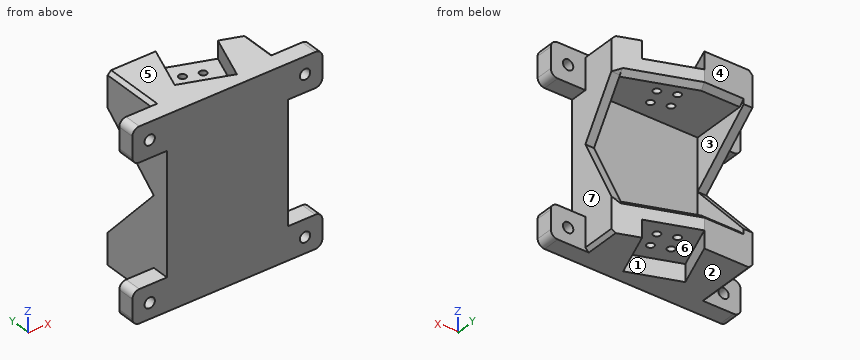
```python
from build123d import *

# Parameters (mm, degrees)
EXTRUDE_1_DEPTH          = 35
EXTRUDE_1_2_DEPTH        = 35
CUT_EXTRUDE_1_DEPTH      = 104.662915259
CUT_EXTRUDE_1_DEPTH_BACK = 104.662915259
SKETCH_2_R               = 2.1
SKETCH_3_W               = 70
SKETCH_3_H               = 10
EXTRUDE_2_DEPTH          = 89
EXTRUDE_3_DEPTH          = 10
EXTRUDE_4_DEPTH          = 10
SKETCH_8_W               = 20
SKETCH_8_H               = 19
SKETCH_8_R               = 3
SKETCH_8_H_2             = 20
EXTRUDE_9_DEPTH          = 10
EXTRUDE_10_DEPTH         = 5
CUT_EXTRUDE_2_DEPTH      = 130.251692445
CUT_EXTRUDE_2_DEPTH_BACK = 130.251692445
EXTRUDE_12_DEPTH         = 5
FILLET_1_R               = 4
FILLET_2_R               = 4
CHAMFER_3_SIZE           = 3
CHAMFER_4_SIZE           = 2


with BuildPart() as part:
    # Sketch 1 → Extrude 1 (new body)
    with BuildSketch(Plane(origin=(0, 0, 0), x_dir=(1, 0, 0), z_dir=(0, 1, 0))):
        Polygon((0, -40), (30, -40), (30, -30), (-40, -30), (-40, -40), align=None)
    extrude(amount=EXTRUDE_1_DEPTH)


with BuildPart() as body_2:
    # Sketch 1 → Extrude 1 2 (new body)
    with BuildSketch(Plane(origin=(0, 0, 0), x_dir=(1, 0, 0), z_dir=(0, 1, 0))):
        Polygon((0, 49), (30, 49), (30, 39), (-40, 39), (-40, 49), align=None)
    extrude(amount=EXTRUDE_1_2_DEPTH)


with BuildPart() as cut_extrude_1_tool:
    # Sketch 2 → Cut-Extrude 1 (new, two sides: drawn at the far end of the back side and taken through both)
    with BuildSketch(Plane.XY.offset(40).offset(-CUT_EXTRUDE_1_DEPTH_BACK)):
        with Locations((0, 10)):
            Circle(SKETCH_2_R)
        with Locations((-9.396926208, 13.420201433)):
            Circle(SKETCH_2_R)
        with Locations((3.420201433, 19.396926208)):
            Circle(SKETCH_2_R)
        with Locations((-5.976724775, 22.817127641)):
            Circle(SKETCH_2_R)
    extrude(amount=CUT_EXTRUDE_1_DEPTH + CUT_EXTRUDE_1_DEPTH_BACK)


with BuildPart() as part_1:
    add(part.part)

    # Cut-Extrude 1: cut by cut_extrude_1_tool
    add(cut_extrude_1_tool.part, mode=Mode.SUBTRACT)



with BuildPart() as body_2_1:
    add(body_2.part)

    # Cut-Extrude 1: cut by cut_extrude_1_tool
    add(cut_extrude_1_tool.part, mode=Mode.SUBTRACT)


with BuildPart() as part_2:
    add(part_1.part)

    add(body_2_1.part)  # Extrude 2 merges body 2
    # Sketch 3 → Extrude 2 (add)
    with BuildSketch(Plane.XY.offset(40)):
        with Locations((-5, -5)):
            Rectangle(SKETCH_3_W, SKETCH_3_H)
    extrude(amount=-EXTRUDE_2_DEPTH)

    # Sketch 4 → Extrude 3 (add)
    with BuildSketch(Plane.XY.offset(40)):
        Polygon((5.976724775, -2.817127641), (-22.214053849, 7.443476659), (-12.184299593, 35), (-40, 35), (-40, -10), (30, -10), (30, 35), (19.741033581, 35), align=None)
    extrude(amount=EXTRUDE_3_DEPTH)

    # Sketch 5 → Extrude 4 (add)
    with BuildSketch(Plane(origin=(0, 0, -49), x_dir=(-1, 0, 0), z_dir=(0, 0, -1))):
        Polygon((-30, 35), (-30, -10), (40, -10), (40, 35), (12.184299593, 35), (22.214053849, 7.443476659), (-5.976724775, -2.817127641), (-19.741033581, 35), align=None)
    extrude(amount=EXTRUDE_4_DEPTH)

    # Sketch 8 → Extrude 9 (add)
    # profile 1 of 4: a face of its own
    with BuildSketch(Plane(origin=(0, -10, 0), x_dir=(-1, 0, 0), z_dir=(0, -1, 0))):
        with Locations((-40, 49.5)):
            Rectangle(SKETCH_8_W, SKETCH_8_H)
        with Locations(Location((-40, 50, 0), (0, 0, 90))):
            Circle(SKETCH_8_R, mode=Mode.SUBTRACT)
    # profile 2 of 4: a face of its own
    with BuildSketch(Plane(origin=(0, -10, 0), x_dir=(-1, 0, 0), z_dir=(0, -1, 0))):
        with Locations((-40, -40)):
            Rectangle(SKETCH_8_W, SKETCH_8_H_2)
        with Locations(Location((-40, -40, 0), (0, 0, 90))):
            Circle(SKETCH_8_R, mode=Mode.SUBTRACT)
    # profile 3 of 4: a face of its own
    with BuildSketch(Plane(origin=(0, -10, 0), x_dir=(-1, 0, 0), z_dir=(0, -1, 0))):
        with Locations((50, 49.5)):
            Rectangle(SKETCH_8_W, SKETCH_8_H)
        with Locations(Location((50, 50, 0), (0, 0, 90))):
            Circle(SKETCH_8_R, mode=Mode.SUBTRACT)
    # profile 4 of 4: a face of its own
    with BuildSketch(Plane(origin=(0, -10, 0), x_dir=(-1, 0, 0), z_dir=(0, -1, 0))):
        with Locations((50, -40)):
            Rectangle(SKETCH_8_W, SKETCH_8_H_2)
        with Locations(Location((50, -40, 0), (0, 0, 90))):
            Circle(SKETCH_8_R, mode=Mode.SUBTRACT)
    extrude(amount=-EXTRUDE_9_DEPTH)

    # Sketch 6 → Extrude 10 (add)
    with BuildSketch(Plane.ZY.offset(40)):
        Polygon((-39, 0), (0, 0), (-39, 35), align=None)
        Polygon((30, 0), (30, 35), (0, 0), align=None)
    extrude(amount=-EXTRUDE_10_DEPTH)

    # Sketch 10 → Cut-Extrude 2 (cut, two sides: drawn at the far end of the back side and taken through both)
    with BuildSketch(Plane.XY.offset(50).offset(-CUT_EXTRUDE_2_DEPTH_BACK)):
        Polygon((30, 19.646170595), (-12.184299593, 35), (30, 35), align=None)
    extrude(amount=CUT_EXTRUDE_2_DEPTH + CUT_EXTRUDE_2_DEPTH_BACK, mode=Mode.SUBTRACT)

    # Sketch 9 → Extrude 12 (add)
    with BuildSketch(Plane(origin=(30, 0, 0), x_dir=(0, 0, -1), z_dir=(1, 0, 0))):
        Polygon((39, 19.646170595), (39, 0), (0, 0), align=None)
        Polygon((0, 0), (-30, 19.646170595), (-30, 0), align=None)
    extrude(amount=-EXTRUDE_12_DEPTH)

    # Fillet 1
    fillet_1_edges = [part_2.edges().sort_by_distance(p)[0] for p in [
        (50, -5, -59),
        (50, -5, 50),
        (-60, -5, -59),
        (-60, -5, 50),
    ]]
    fillet(fillet_1_edges, radius=FILLET_1_R)

    # Fillet 2
    fillet_2_edges = [part_2.edges().sort_by_distance(p)[0] for p in [
        (50, -5, -40),
        (50, -5, 30),
        (-60, -5, -40),
        (-60, -5, 30),
    ]]
    fillet(fillet_2_edges, radius=FILLET_2_R)

    # Chamfer 3
    # the kernel refuses this chamfer: 3 mm, written as the material it takes off along each edge
    with BuildSketch(Plane(origin=(-4.469250629, 35, -39), x_dir=(0, 0.027495876610586768, -0.9996219169112968), z_dir=(-1, 0, 0))) as chamfer_3_piece_1:
        Polygon((CHAMFER_3_SIZE * 0.999621916911, CHAMFER_3_SIZE * 0.0274958766106), (-CHAMFER_3_SIZE * 0.0274958766106, CHAMFER_3_SIZE * 0.999621916911), (0, 0), align=None)
    extrude(amount=30.530749371, mode=Mode.SUBTRACT)
    with BuildSketch(Plane(origin=(-19.434074173, 37.638702152, -39), x_dir=(0.009404143659217951, 0.02583767235300856, -0.9996219169112968), z_dir=(0.9396926207859079, -0.34202014332567027, 0))) as chamfer_3_piece_2_section:
        Polygon((CHAMFER_3_SIZE * 0.999621916911, -CHAMFER_3_SIZE * 0.0274958766106), (-CHAMFER_3_SIZE * 0.0274958766106, -CHAMFER_3_SIZE * 0.999621916911), (0, 0), align=None)
    chamfer_3_piece_2 = extrude(amount=60.321691902, mode=Mode.PRIVATE)
    chamfer_3_piece_2 = split(chamfer_3_piece_2, bisect_by=Plane(origin=(25, 27.771188546, -39.985901666), z_dir=(-1, 0, 0)), keep=Keep.TOP, mode=Mode.PRIVATE)
    add(chamfer_3_piece_2, mode=Mode.SUBTRACT)
    with BuildSketch(Plane(origin=(-19.434074173, 37.638702152, -39), x_dir=(0.009404143659217951, 0.02583767235300856, -0.9996219169112968), z_dir=(0.9396926207859079, -0.34202014332567027, 0))) as chamfer_3_piece_3_section:
        Polygon((CHAMFER_3_SIZE * 0.999621916911, -CHAMFER_3_SIZE * 0.0274958766106), (-CHAMFER_3_SIZE * 0.0274958766106, -CHAMFER_3_SIZE * 0.999621916911), (0, 0), align=None)
    chamfer_3_piece_3 = extrude(amount=60.321691902, mode=Mode.PRIVATE)
    chamfer_3_piece_3 = split(chamfer_3_piece_3, bisect_by=Plane(origin=(26.25970181, 20.183987428, -40.067630782), z_dir=(0, 0.8930842834154016, 0.4498893894241103)), keep=Keep.TOP, mode=Mode.PRIVATE)
    add(chamfer_3_piece_3, mode=Mode.SUBTRACT)
    with BuildSketch(Plane(origin=(-4.469250629, 35, 30), x_dir=(0, 0.027495876610586768, 0.9996219169112968), z_dir=(-1, 0, 0))) as chamfer_3_piece_4:
        Polygon((CHAMFER_3_SIZE * 0.999621916911, -CHAMFER_3_SIZE * 0.0274958766106), (-CHAMFER_3_SIZE * 0.0274958766106, -CHAMFER_3_SIZE * 0.999621916911), (0, 0), align=None)
    extrude(amount=30.530749371, mode=Mode.SUBTRACT)
    with BuildSketch(Plane(origin=(-19.434074173, 37.638702152, 30), x_dir=(0.009404143659217682, 0.025837672353007816, 0.9996219169112968), z_dir=(0.9396926207859079, -0.34202014332567027, 0))) as chamfer_3_piece_5_section:
        Polygon((CHAMFER_3_SIZE * 0.999621916911, CHAMFER_3_SIZE * 0.0274958766106), (-CHAMFER_3_SIZE * 0.0274958766106, CHAMFER_3_SIZE * 0.999621916911), (0, 0), align=None)
    chamfer_3_piece_5 = extrude(amount=60.321691902, mode=Mode.PRIVATE)
    chamfer_3_piece_5 = split(chamfer_3_piece_5, bisect_by=Plane(origin=(25, 27.800984408, 30.984043991), z_dir=(-1, 0, 0)), keep=Keep.TOP, mode=Mode.PRIVATE)
    add(chamfer_3_piece_5, mode=Mode.SUBTRACT)
    with BuildSketch(Plane(origin=(-19.434074173, 37.638702152, 30), x_dir=(0.009404143659217682, 0.025837672353007816, 0.9996219169112968), z_dir=(0.9396926207859079, -0.34202014332567027, 0))) as chamfer_3_piece_6_section:
        Polygon((CHAMFER_3_SIZE * 0.999621916911, CHAMFER_3_SIZE * 0.0274958766106), (-CHAMFER_3_SIZE * 0.0274958766106, CHAMFER_3_SIZE * 0.999621916911), (0, 0), align=None)
    chamfer_3_piece_6 = extrude(amount=60.321691902, mode=Mode.PRIVATE)
    chamfer_3_piece_6 = split(chamfer_3_piece_6, bisect_by=Plane(origin=(26.25, 20.237686054, 30.903253063), z_dir=(0, 0.8365761810170901, -0.547850612261099)), keep=Keep.TOP, mode=Mode.PRIVATE)
    add(chamfer_3_piece_6, mode=Mode.SUBTRACT)

    # Chamfer 4
    chamfer_4_edges = [part_2.edges().sort_by_distance(p)[0] for p in [
        (30, 9.823085297, 50),
        (-40, 17.5, -59),
        (30, 9.823085297, -59),
        (-40, 17.5, 50),
    ]]
    chamfer(chamfer_4_edges, length=CHAMFER_4_SIZE)


solid = part_2.part
```
For this review, take the finished solid that the model builds, in its own axes (mm). Face numbers are marked on the shaded views. A direction names the side the tool comes from. Round coordinates to 2 decimals unless told otherwise and drop trailing zeros. Loops run counter-clockwise (first coordinate to the right, second up) from the corner with the lowest first, then second, coordinate; pieces in that order, holes last.
Q1. Add section C-C on x = -27. Write out the cut boundary in (y, z).
Result sheet:
outline: (-10, -59) - (35, -59) - (35, -42) - (32, -39) - (0, -39) - (0, 30) - (32, 30) - (35, 33) - (35, 50) - (-10, 50) - close
Q2. Mouldability with a two-part tool opening along Z and no side actions: class the marked faces 4, 5, 6 and 7 as +Z half, -Z half, draft (parallel to the pull), parting line (faces both ways), or undercut.
Result sheet:
face 4: draft
face 5: +Z half
face 6: -Z half
face 7: undercut
Q3. Machinability: for the marked faces 1, 2 and 3, which of the approach directions +Z, -Z, +X, -X, +Y, -Y give a long, thin tool a straight path to every point of the face, cutting with its end or side? Answer none if there is none.
Result sheet:
face 1: -Z
face 2: -Z, +X, -X, +Y, -Y
face 3: +Y
Q4. To check wall thickness, follow line 1 along X through (y, z) = (-5, -50); line 2 along X through (y, z) = (7.5, 12.5); line 3 along Z through (x, y) = (0, 17). State the ranges of each line that lie inside material, in increasing order.
Result sheet:
line 1: x = -60 to -53, -47 to 37, 43 to 50
line 2: x = -40 to -35, 25 to 30
line 3: z = -49 to -39, 30 to 40
Q5. Add section B-B on y = -6. Write out the cut boundary in (x, z).
Result sheet:
outline: (-60, -55) arc R4 ccw to (-56, -59) - (46, -59) arc R4 ccw to (50, -55) - (50, -44) arc R4 ccw to (46, -40) - (30, -40) - (30, 30) - (46, 30) arc R4 ccw to (50, 34) - (50, 46) arc R4 ccw to (46, 50) - (-56, 50) arc R4 ccw to (-60, 46) - (-60, 34) arc R4 ccw to (-56, 30) - (-40, 30) - (-40, -40) - (-56, -40) arc R4 ccw to (-60, -44) - close; hole circle Ø6 at (-50, -50); hole circle Ø6 at (-50, 40); hole circle Ø6 at (40, -50); hole circle Ø6 at (40, 40)
Q6. Add section D-D on z = -30. Write out the cut boundary in (x, y).
Result sheet:
outline: (-40, -10) - (30, -10) - (30, 15.11) - (25, 15.11) - (25, 0) - (-35, 0) - (-35, 26.92) - (-40, 26.92) - close
Q7. Insertion check: pin 1 Ø10 at (y, z) = (8.5, -3) entering from +X; pin 2 Ø5 at (x, z) = (40, 40) entering from -Y; pin 3 Ø4 at (x, y) = (-0.5, 21.5) entering from -Z; pin 4 Ø9.5 at (x, z) = (35.5, -53.5) entering from +Y. Each pin has a flat end and moves straight along its axis. Give the tip position at first contact, or say it passes through.
Result sheet:
pin 1: stops at x = -35
pin 2: passes through
pin 3: stops at z = -49
pin 4: stops at y = 0
Q8. Add section A-A on x = -50. Write out the cut boundary in (y, z).
Result sheet:
outline: (-10, -59) - (0, -59) - (0, -53) - (-10, -53) - close; (-10, -47) - (0, -47) - (0, -40) - (-10, -40) - close; (-10, 30) - (0, 30) - (0, 37) - (-10, 37) - close; (-10, 43) - (0, 43) - (0, 50) - (-10, 50) - close
